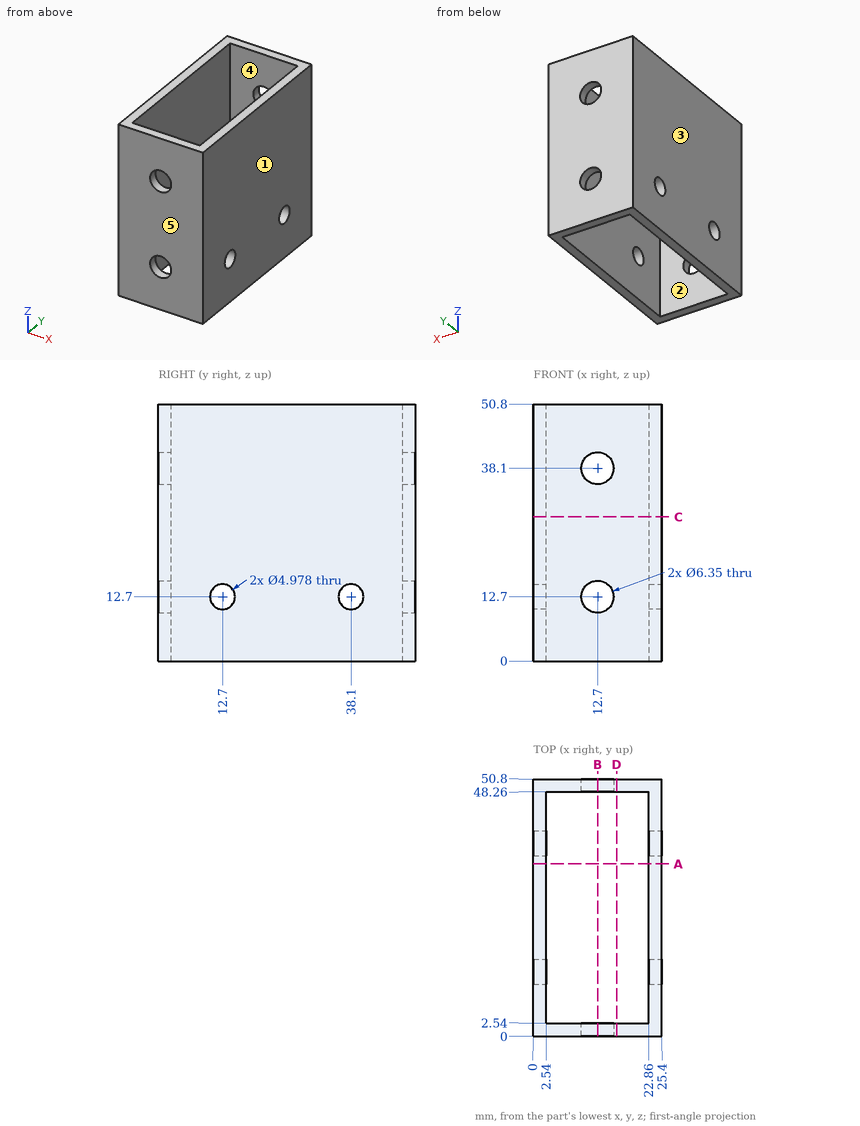
Job drawing, mm, ordinate dimensions from the low corner. One solid piece. A direction names the side the tool comes from. Coordinates: 2 decimals unless noted, no trailing zeros. Write each loop counter-clockwise with the first axis right and the second up, starting at its lowest first coordinate (ties: lowest second). Pieces come first, ordered by that corner, then holes.
Item 1: Probe line 1 (Y direction, x = 2, z = 12.7); line 2 (Y direction, x = 10.5, z = 23); line 3 (X direction, y = 1, z = 12.7) (1 decimal). List the from-to ranges inside material, lowest first.
Item 2: Slice it at D-D (x = 16.5). Write the cut outline in (y, z).
Item 3: Slice it at A-A (y = 34). Write the cut outline in (x, z), and give its area (3 significant figures).
Item 4: Which spindle directions (+Z, -Z, +X, -X, +Y, -Y) get a long thin tool onto all of the face, cutting with end or side? Do the marked faces 4 and 5. Say none if no direction does.
Item 5: Pin check, flat tip, straight feed: pin 1 (5.5 mm diameter, centred on x = 12.7, z = 38.1, fed in from +Y). Stop position of the tip, or through.
Item 6: Mould opens along X. For the marked faces 1, 2 and 3 say: released by +X, released by -X, zero draft, split by the parting line, or undercut.
Item 7: Slice it at B-B (x = 12.7). Write the cut outline in (y, z) (1 decimal).
Item 8: Slice it at C-C (z = 28.5). Write the cut outline in (x, y).
Results found:
1. line 1: y = 0 to 10.21, 15.19 to 35.61, 40.59 to 50.8
1. line 2: y = 0 to 2.54, 48.26 to 50.8
1. line 3: x = 0 to 9.5, 15.9 to 25.4
2. outline: (0, 0) - (2.54, 0) - (2.54, 50.8) - (0, 50.8) - close; (48.26, 0) - (50.8, 0) - (50.8, 50.8) - (48.26, 50.8) - close
3. outline: (0, 0) - (2.54, 0) - (2.54, 50.8) - (0, 50.8) - close; (22.86, 0) - (25.4, 0) - (25.4, 50.8) - (22.86, 50.8) - close
3. area: 258 mm2
4. face 4: +Z, -Z
4. face 5: +Z, -Z, +X, -X, -Y
5. pin 1: passes through
6. face 1: released by +X
6. face 2: undercut
6. face 3: released by -X
7. outline: (0, 0) - (2.5, 0) - (2.5, 9.5) - (0, 9.5) - close; (0, 15.9) - (2.5, 15.9) - (2.5, 34.9) - (0, 34.9) - close; (0, 41.3) - (2.5, 41.3) - (2.5, 50.8) - (0, 50.8) - close; (48.3, 0) - (50.8, 0) - (50.8, 9.5) - (48.3, 9.5) - close; (48.3, 15.9) - (50.8, 15.9) - (50.8, 34.9) - (48.3, 34.9) - close; (48.3, 41.3) - (50.8, 41.3) - (50.8, 50.8) - (48.3, 50.8) - close
8. outline: (0, 0) - (25.4, 0) - (25.4, 50.8) - (0, 50.8) - close; hole (2.54, 2.54) - (22.86, 2.54) - (22.86, 48.26) - (2.54, 48.26) - close
